```python
from build123d import *

# Parameters (mm, degrees)
BOSS_EXTRUDE1_DEPTH = 25
FILLET1_R           = 5
SKETCH2_R           = 5
CUT_EXTRUDE1_DEPTH  = 137.839321834
SKETCH3_R           = 5
CUT_EXTRUDE2_DEPTH  = 137.839321834


with BuildPart() as part:
    # Sketch1 → Boss-Extrude1 (new, symmetric)
    with BuildSketch(Plane(origin=(0, 0, 0), x_dir=(1, 0, 0), z_dir=(0, 1, 0))):
        Polygon((0, 0), (0, 100), (10, 100), (10, 10), (100, 10), (100, 0), align=None)
    extrude(amount=BOSS_EXTRUDE1_DEPTH, both=True)

    # Fillet1
    fillet1_edges = [part.edges().sort_by_distance(p)[0] for p in [
        (10, 0, -10),
    ]]
    fillet(fillet1_edges, radius=FILLET1_R)

    # Sketch2 → Cut-Extrude1 (cut, through all)
    with BuildSketch(Plane(origin=(10, 0, 0), x_dir=(0, 0, -1), z_dir=(1, 0, 0))):
        with Locations((33.333, 0)):
            Circle(SKETCH2_R)
        with Locations((66.666, 0)):
            Circle(SKETCH2_R)
    extrude(amount=-CUT_EXTRUDE1_DEPTH, mode=Mode.SUBTRACT)

    # Sketch3 → Cut-Extrude2 (cut, through all)
    with BuildSketch(Plane(origin=(0, 0, -10), x_dir=(-1, 0, 0), z_dir=(0, 0, -1))):
        with Locations((-33.33, 0)):
            Circle(SKETCH3_R)
        with Locations((-66.66, 0)):
            Circle(SKETCH3_R)
    extrude(amount=-CUT_EXTRUDE2_DEPTH, mode=Mode.SUBTRACT)


solid = part.part
```
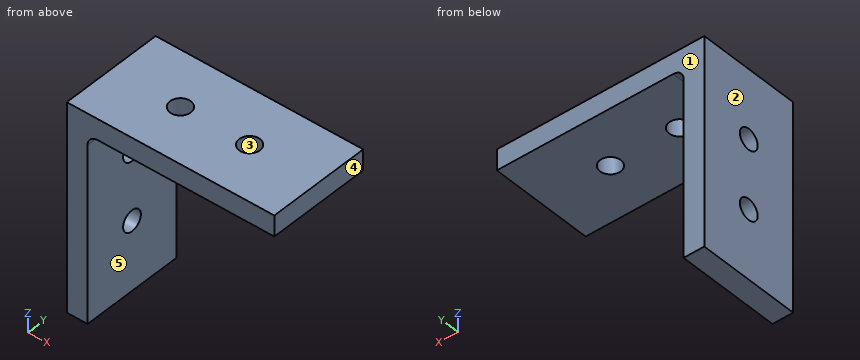
Check sheet for the modelled part. Datum: model origin and axes. Units: mm. Face numbers are marked on the shaded views. A direction names the side the tool comes from. Give positions to 0.01 mm unless a question says otherwise; leave off trailing zeros. Loops run counter-clockwise (first coordinate to the right, second up) from the corner with the lowest first, then second, coordinate; pieces in that order, holes last. Notation, with made-up numbers: (18.25, 87) - (52.25, 87) arc R36 ccw to (52.25, 121) - close; hole circle Ø9 at (1, -17.75). An arc over 180 degrees is marked (long way). One line per question, with ' | ' between items. Start each with the question number.
1. Material ranges on line 1 along Y through (x, z) = (66.66, -6.5); line 2 along X through (y, z) = (17, -65); line 3 along Z through (x, y) = (30, -12.5), recorded low to high. Write a range as [from, to].
2. Draft check along Y on the marked faces 1, 2 and 3. Enter one of: released by +Y, released by -Y, zero draft, split by the parting line, or undercut.
3. Set-up check for the marked faces 4 and 5: record each of +Z, -Z, +X, -X, +Y, -Y from which the full face is reachable in a straight line by a thin tool's end or side.
4. Cross-section at B-B, the plane y = 0. Enter the section's corners in (x, z).
5. Cross-section at D-D, the plane y = 19.5. Enter the section's corners in (x, z).
6. Gauge pin test, flat ends, axial feed: pin 1 Ø9 at (y, z) = (0, -66.666) entering from +X; pin 2 Ø15 at (x, y) = (39.5, 7) entering from -Z. Record the tip position at first contact, or that the pin passes through.
7. Cross-section at C-C, the plane z = -37. Enter the section's corners in (x, y), plus the area to 3 significant figures.
8. Cross-section at A-A, the plane x = 33.33. Enter the section's corners in (y, z).
Check result:
1) line 1: y = [-25, -5], [5, 25] | line 2: x = [0, 10] | line 3: z = [-10, 0]
2) face 1: released by +Y | face 2: zero draft | face 3: undercut
3) face 4: +Z, -Z, +X, +Y, -Y | face 5: -Z, +X, +Y, -Y
4) outline: (0, -100) - (10, -100) - (10, -71.67) - (0, -71.67) - close; (0, -61.67) - (10, -61.67) - (10, -38.33) - (0, -38.33) - close; (0, -28.33) - (10, -28.33) - (10, -15) arc R5 cw to (15, -10) - (28.33, -10) - (28.33, 0) - (0, 0) - close; (38.33, -10) - (61.66, -10) - (61.66, 0) - (38.33, 0) - close; (71.66, -10) - (100, -10) - (100, 0) - (71.66, 0) - close
5) outline: (0, -100) - (10, -100) - (10, -15) arc R5 cw to (15, -10) - (100, -10) - (100, 0) - (0, 0) - close
6) pin 1: passes through | pin 2: stops at z = -10
7) outline: (0, -25) - (10, -25) - (10, -3.4) - (0, -3.4) - close; (0, 3.4) - (10, 3.4) - (10, 25) - (0, 25) - close | area: 432 mm2
8) outline: (-25, -10) - (-5, -10) - (-5, 0) - (-25, 0) - close; (5, -10) - (25, -10) - (25, 0) - (5, 0) - close
